Can you work these out from the model? Positions are in its coordinate system, mm. Round coordinates to 2 decimals unless told otherwise and drop trailing zeros. Loops run counter-clockwise (first coordinate to the right, second up) from the corner with the lowest first, then second, coordinate; pieces in that order, holes last. Notation, with made-up numbers: M 28.25,29 L 66.25,29 A30 ccw 66.25,62 Z; hole C 74,-33.5 d7. An arc over 180 degrees is marked long. Return JSON: item names as keys, results as strings.
```python
from build123d import *

# Parameters (mm, degrees)
SKETCH1_W           = 914.4
SKETCH1_H           = 304.8
BOSS_EXTRUDE1_DEPTH = 12.7
SKETCH5_W           = 609.6
SKETCH5_H           = 38.1
CUT_EXTRUDE3_DEPTH  = 2.54
SKETCH6_R           = 46.99
CUT_EXTRUDE4_DEPTH  = 964.945895785
SKETCH7_R           = 63.5
CUT_EXTRUDE5_DEPTH  = 7.62
CUT_EXTRUDE6_DEPTH  = 964.945895785
CUT_EXTRUDE7_DEPTH  = 3.175
SKETCH13_W          = 19.05
SKETCH13_H          = 19.05
CUT_EXTRUDE11_DEPTH = 964.945895785
CUT_EXTRUDE19_DEPTH = 964.945895785
CUT_EXTRUDE20_DEPTH = 2.54
SKETCH26_R          = 3.302
CUT_EXTRUDE21_DEPTH = 964.945895785
SKETCH19_W          = 914.4
SKETCH19_H          = 304.8
CUT_EXTRUDE16_DEPTH = 6.35


with BuildPart() as part:
    # Sketch1 → Boss-Extrude1 (new body)
    with BuildSketch(Plane(origin=(0, 0, 0), x_dir=(1, 0, 0), z_dir=(0, 1, 0))):
        with Locations((457.2, 152.4)):
            Rectangle(SKETCH1_W, SKETCH1_H)
    extrude(amount=BOSS_EXTRUDE1_DEPTH)

    # Sketch5 → Cut-Extrude3 (cut)
    with BuildSketch(Plane(origin=(0, 12.7, 0), x_dir=(1, 0, 0), z_dir=(0, 1, 0))):
        with Locations((508, 88.9)):
            Rectangle(SKETCH5_W, SKETCH5_H)
    extrude(amount=-CUT_EXTRUDE3_DEPTH, mode=Mode.SUBTRACT)

    # Sketch6 → Cut-Extrude4 (cut, through all)
    with BuildSketch(Plane(origin=(0, 12.7, 0), x_dir=(1, 0, 0), z_dir=(0, 1, 0))):
        with Locations(Location((82.55, 222.25, 0), (0, 0, 270))):
            Circle(SKETCH6_R)
        with Locations(Location((831.85, 222.25, 0), (0, 0, 270))):
            Circle(SKETCH6_R)
    extrude(amount=-CUT_EXTRUDE4_DEPTH, mode=Mode.SUBTRACT)

    # Sketch7 → Cut-Extrude5 (cut)
    with BuildSketch(Plane(origin=(0, 12.7, 0), x_dir=(1, 0, 0), z_dir=(0, 1, 0))):
        with Locations(Location((82.55, 222.25, 0), (0, 0, 270))):
            Circle(SKETCH7_R)
        with Locations(Location((831.85, 222.25, 0), (0, 0, 270))):
            Circle(SKETCH7_R)
    extrude(amount=-CUT_EXTRUDE5_DEPTH, mode=Mode.SUBTRACT)

    # Sketch8 → Cut-Extrude6 (cut, through all)
    with BuildSketch(Plane(origin=(0, 12.7, 0), x_dir=(1, 0, 0), z_dir=(0, 1, 0))):
        with BuildLine():
            Line((381, 285.75), (381, 209.55))
            ThreePointArc((381, 209.55), (382.859871939, 205.059871939), (387.35, 203.2))
            Line((387.35, 203.2), (527.05, 203.2))
            ThreePointArc((527.05, 203.2), (531.540128061, 205.059871939), (533.4, 209.55))
            Line((533.4, 209.55), (533.4, 285.75))
            ThreePointArc((533.4, 285.75), (531.540128061, 290.240128061), (527.05, 292.1))
            Line((527.05, 292.1), (387.35, 292.1))
            ThreePointArc((387.35, 292.1), (382.859871939, 290.240128061), (381, 285.75))
        make_face()
    extrude(amount=-CUT_EXTRUDE6_DEPTH, mode=Mode.SUBTRACT)

    # Sketch9 → Cut-Extrude7 (cut)
    with BuildSketch(Plane(origin=(0, 12.7, 0), x_dir=(1, 0, 0), z_dir=(0, 1, 0))):
        with BuildLine():
            Line((539.75, 304.8), (374.65, 304.8))
            Line((374.65, 304.8), (374.65, 202.946))
            ThreePointArc((374.65, 202.946), (376.509871939, 198.455871939), (381, 196.596))
            Line((381, 196.596), (533.4, 196.596))
            ThreePointArc((533.4, 196.596), (537.890128061, 198.455871939), (539.75, 202.946))
            Line((539.75, 202.946), (539.75, 304.8))
        make_face()
    extrude(amount=-CUT_EXTRUDE7_DEPTH, mode=Mode.SUBTRACT)

    # Sketch13 → Cut-Extrude11 (cut, through all)
    with BuildSketch(Plane(origin=(0, 12.7, 0), x_dir=(1, 0, 0), z_dir=(0, 1, 0))):
        with Locations((47.625, 117.475)):
            Rectangle(SKETCH13_W, SKETCH13_H)
        with Locations((76.2, 117.475)):
            Rectangle(SKETCH13_W, SKETCH13_H)
    extrude(amount=-CUT_EXTRUDE11_DEPTH, mode=Mode.SUBTRACT)

    # Sketch24 → Cut-Extrude19 (cut, through all)
    with BuildSketch(Plane(origin=(0, 12.7, 0), x_dir=(1, 0, 0), z_dir=(0, 1, 0))):
        with BuildLine():
            Line((111.125, 127), (179.3875, 127))
            ThreePointArc((179.3875, 127), (183.877628061, 125.140128061), (185.7375, 120.65))
            Line((185.7375, 120.65), (185.7375, 25.4))
            ThreePointArc((185.7375, 25.4), (183.877628061, 20.909871939), (179.3875, 19.05))
            Line((179.3875, 19.05), (111.125, 19.05))
            ThreePointArc((111.125, 19.05), (106.634871939, 20.909871939), (104.775, 25.4))
            Line((104.775, 25.4), (104.775, 120.65))
            ThreePointArc((104.775, 120.65), (106.634871939, 125.140128061), (111.125, 127))
        make_face()
    extrude(amount=-CUT_EXTRUDE19_DEPTH, mode=Mode.SUBTRACT)

    # Sketch25 → Cut-Extrude20 (cut)
    with BuildSketch(Plane(origin=(0, 12.7, 0), x_dir=(1, 0, 0), z_dir=(0, 1, 0))):
        with BuildLine():
            Line((104.775, 133.35), (185.7375, 133.35))
            ThreePointArc((185.7375, 133.35), (190.227628061, 131.490128061), (192.0875, 127))
            Line((192.0875, 127), (192.0875, 19.05))
            ThreePointArc((192.0875, 19.05), (190.227628061, 14.559871939), (185.7375, 12.7))
            Line((185.7375, 12.7), (104.775, 12.7))
            ThreePointArc((104.775, 12.7), (100.284871939, 14.559871939), (98.425, 19.05))
            Line((98.425, 19.05), (98.425, 127))
            ThreePointArc((98.425, 127), (100.284871939, 131.490128061), (104.775, 133.35))
        make_face()
    extrude(amount=-CUT_EXTRUDE20_DEPTH, mode=Mode.SUBTRACT)

    # Sketch26 → Cut-Extrude21 (cut, through all)
    with BuildSketch(Plane(origin=(0, 12.7, 0), x_dir=(1, 0, 0), z_dir=(0, 1, 0))):
        with Locations(Location((863.6, 107.95, 0), (0, 0, 270))):
            Circle(SKETCH26_R)
    extrude(amount=-CUT_EXTRUDE21_DEPTH, mode=Mode.SUBTRACT)

    # Sketch19 → Cut-Extrude16 (cut)
    with BuildSketch(Plane.XZ):
        with Locations((457.2, -152.4)):
            Rectangle(SKETCH19_W, SKETCH19_H)
        with BuildLine():
            Line((12.7, -139.7), (12.7, -292.1))
            Line((12.7, -292.1), (317.5, -292.1))
            Line((317.5, -292.1), (317.5, -146.05))
            ThreePointArc((317.5, -146.05), (315.640128061, -141.559871939), (311.15, -139.7))
            Line((311.15, -139.7), (12.7, -139.7))
        make_face(mode=Mode.SUBTRACT)
        with BuildLine():
            Line((596.9, -292.1), (901.7, -292.1))
            Line((901.7, -292.1), (901.7, -139.7))
            Line((901.7, -139.7), (603.25, -139.7))
            ThreePointArc((603.25, -139.7), (598.759871939, -141.559871939), (596.9, -146.05))
            Line((596.9, -146.05), (596.9, -292.1))
        make_face(mode=Mode.SUBTRACT)
        with BuildLine():
            Line((12.7, -127), (12.7, -12.7))
            Line((12.7, -12.7), (901.7, -12.7))
            Line((901.7, -12.7), (901.7, -127))
            Line((901.7, -127), (590.55, -127))
            ThreePointArc((590.55, -127), (586.059871939, -128.859871939), (584.2, -133.35))
            Line((584.2, -133.35), (584.2, -292.1))
            Line((584.2, -292.1), (330.2, -292.1))
            Line((330.2, -292.1), (330.2, -133.35))
            ThreePointArc((330.2, -133.35), (328.340128061, -128.859871939), (323.85, -127))
            Line((323.85, -127), (12.7, -127))
        make_face(mode=Mode.SUBTRACT)
    extrude(amount=-CUT_EXTRUDE16_DEPTH, mode=Mode.SUBTRACT)


solid = part.part
```
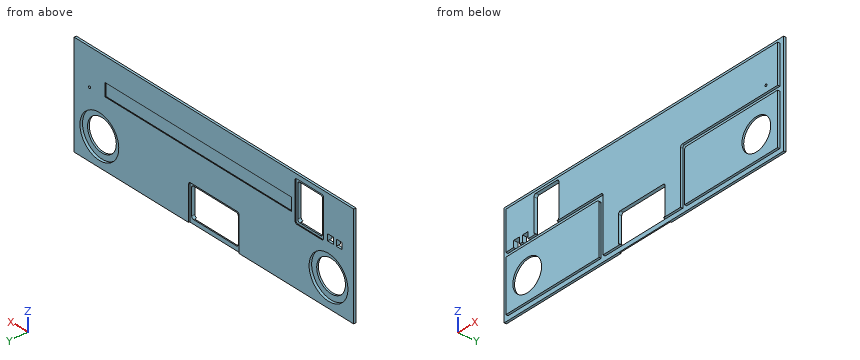
Q1. Suppose I cut it at D-D, the plane z = -222.25. State how many separate pieces and enclosed holes the cut face has, plus the area to 3 significant figures.
Results:
{"separate pieces": "4", "enclosed holes": "0", "area": "6,420 mm2"}
Q2. I'm going to push flat-ended pins straight in: pin 1 Ø2.5 at (x, y) = (460, 11.5) entering from -Z; pin 2 Ø3 at (x, y) = (21.5, 4.5) entering from -Z; pin 3 Ø0.8 at (x, y) = (137, 11) entering from +Z; pin 4 Ø7 at (y, z) = (2, -228.5) entering from -X. Where does each tip first touch, or does it pass through?
Results:
{"pin 1": "stops at z = -196.6", "pin 2": "stops at z = -292.1", "pin 3": "stops at z = 0", "pin 4": "stops at x = 12.7"}
Q3. Suppose I cut it at B-B, the plane x = 721.5. Please give me the cut outline in (y, z), plus the area to 3 significant figures.
Results:
{"outline": "M 0,-292.1 L 6.35,-292.1 L 6.35,-304.8 L 12.7,-304.8 L 12.7,-107.95 L 10.16,-107.95 L 10.16,-69.85 L 12.7,-69.85 L 12.7,0 L 6.35,0 L 6.35,-12.7 L 0,-12.7 L 0,-127 L 6.35,-127 L 6.35,-139.7 L 0,-139.7 Z", "area": "3,530 mm2"}
Q4. If I drill on line 1 along X through (y, z) = (2.1, -222.25); line 2 along Z through (x, y) = (751.5, 6); line 3 along Z through (x, y) = (836.5, 5), over which ranges is the centre line in solid material (lowest first)?
Results:
{"line 1": "x = 12.7 to 35.56, 129.54 to 317.5, 330.2 to 381, 533.4 to 584.2, 596.9 to 784.86, 878.84 to 901.7", "line 2": "z = -292.1 to -139.7, -127 to -12.7", "line 3": "z = -292.1 to -269.01, -175.49 to -139.7, -127 to -12.7"}
